Here's how the part is built. I have some questions about the finished solid (model axes, mm). A direction names the side the tool comes from. Coordinates: 2 decimals unless noted, no trailing zeros. Order: outer loops, then holes, each group sorted by start corner. A loop starts at its lowest first (then second) coordinate and runs counter-clockwise, first axis right, second up. Notation, with made-up numbers: (30, 12.5) - (70, 12.5) arc R21 ccw to (70, 24.5) - close; hole circle Ø11 at (-11, 34). An arc over 180 degrees is marked (long way). Answer as CSV lines item,"result". Start each with the question number.
Q1. Suppose I cut it at B-B (y = 9). Please give me the cut outline in (x, z).
Q2. Suppose I cut it at A-A (z = 29.5). Please give me the cut outline in (x, y).
Q3. Thinking about a two-plate mould opening in Z: for faces 3 (the face through (-12.545, -5, 19)), 4 (the face through (-13.559, 13.954, 35.976)), 5 (the face through (24.469, 13.954, 38.024)), 6 (the face through (5, -27, 3)), which applies, released by +Z, released by -Z, zero draft, split by the parting line, or undercut?
Q4. For pin 1 Ø1.2 at (y, z) = (-25.09, 37) entering from +X; pin 2 Ø2 at (x, y) = (5, -27) entering from +Z; pin 3 Ø11 at (x, y) = (14.5, -1) entering from +Z; pin 4 Ø4 at (x, z) = (0.5, 1) entering from +Y, each with a flat end and sliding along its axis, tell me the tip position at first contact or that it passes through.
Q5. Suppose I cut it at C-C (x = 19). Please give me the cut outline in (y, z).
Q6. For faces 1 (the face through (7, 16.909, -3)), 2 (the face through (5, -4, -2)), which set-ups out of +Z, -Z, +X, -X, +Y, -Y let a thin tool reach every point of the face, with its end or its side?
Q7. I need wall thicknesses on line 1 (Y direction, x = 24.6, z = 37); line 2 (X direction, y = 10, z = 22.5); line 3 (Z direction, x = 2.5, y = -15.5). Which ranges of each line are inside material? Lowest first, please.
from build123d import *

# Parameters (mm, degrees)
SKETCH_1_W           = 40
SKETCH_1_H           = 45
EXTRUDE_1_DEPTH      = 40
EXTRUDE_1_DEPTH_BACK = 5
SKETCH_2_W           = 36
SKETCH_2_H           = 37
CUT_EXTRUDE_1_DEPTH  = 50
SKETCH_3_R           = 1.025
CUT_EXTRUDE_2_DEPTH  = 2
SKETCH_4_R           = 1.025
CUT_EXTRUDE_3_DEPTH  = 2
SKETCH_5_W           = 36
SKETCH_5_H           = 5
CUT_EXTRUDE_4_DEPTH  = 43
FILLET_6_R           = 5
FILLET_7_R           = 5
FILLET_12_R          = 3
FILLET_13_R          = 3
FILLET_14_R          = 3
FILLET_15_R          = 3


with BuildPart() as part:
    # 草圖1 → 填料-伸長1 (new body, two sides)
    with BuildSketch(Plane.XY) as extrude_1_sk:
        with Locations((5.454545455, -5.590909091)):
            Rectangle(SKETCH_1_W, SKETCH_1_H)
    extrude(amount=EXTRUDE_1_DEPTH)
    extrude(extrude_1_sk.sketch, amount=-EXTRUDE_1_DEPTH_BACK)

    # 草圖2 → 除料-伸長1 (cut)
    with BuildSketch(Plane(origin=(0, 16.909090909, 0), x_dir=(1, 0, 0), z_dir=(0, 1, 0))):
        with Locations((5.454545455, -21.5)):
            Rectangle(SKETCH_2_W, SKETCH_2_H)
    extrude(amount=-CUT_EXTRUDE_1_DEPTH, mode=Mode.SUBTRACT)

    # 草圖3 → 除料-伸長2 (cut)
    with BuildSketch(Plane.ZY.offset(14.545454545)):
        with Locations((37, -25.090909091)):
            Circle(SKETCH_3_R)
        with Locations((37, 13.909090909)):
            Circle(SKETCH_3_R)
    extrude(amount=-CUT_EXTRUDE_2_DEPTH, mode=Mode.SUBTRACT)

    # 草圖4 → 除料-伸長3 (cut)
    with BuildSketch(Plane(origin=(25.454545455, 0, 0), x_dir=(0, 0, -1), z_dir=(1, 0, 0))):
        with Locations((-37, 13.909090909)):
            Circle(SKETCH_4_R)
        with Locations((-37, -25.090909091)):
            Circle(SKETCH_4_R)
    extrude(amount=-CUT_EXTRUDE_3_DEPTH, mode=Mode.SUBTRACT)

    # 草圖5 → 除料-伸長4 (cut)
    with BuildSketch(Plane(origin=(0, 16.909090909, 0), x_dir=(1, 0, 0), z_dir=(0, 1, 0))):
        with Locations((5.454545455, -0.5)):
            Rectangle(SKETCH_5_W, SKETCH_5_H)
    extrude(amount=-CUT_EXTRUDE_4_DEPTH, mode=Mode.SUBTRACT)

    # 圓角6
    fillet_6_edges = [part.edges().sort_by_distance(p)[0] for p in [
        (-14.545454545, -5.590909091, -5),
    ]]
    fillet(fillet_6_edges, radius=FILLET_6_R)

    # 圓角7
    fillet_7_edges = [part.edges().sort_by_distance(p)[0] for p in [
        (25.454545455, -5.590909091, -5),
    ]]
    fillet(fillet_7_edges, radius=FILLET_7_R)

    # 圓角12
    fillet_12_edges = [part.edges().sort_by_distance(p)[0] for p in [
        (-13.545454545, -28.090909091, 40),
    ]]
    fillet(fillet_12_edges, radius=FILLET_12_R)

    # 圓角13
    fillet_13_edges = [part.edges().sort_by_distance(p)[0] for p in [
        (24.454545455, -28.090909091, 40),
    ]]
    fillet(fillet_13_edges, radius=FILLET_13_R)

    # 圓角14
    fillet_14_edges = [part.edges().sort_by_distance(p)[0] for p in [
        (-13.545454545, 16.909090909, 40),
    ]]
    fillet(fillet_14_edges, radius=FILLET_14_R)

    # 圓角15
    fillet_15_edges = [part.edges().sort_by_distance(p)[0] for p in [
        (24.454545455, 16.909090909, 40),
    ]]
    fillet(fillet_15_edges, radius=FILLET_15_R)


solid = part.part
Here are the results:
1,outline,"(-14.55, 0) arc R5 ccw to (-9.55, -5) - (20.45, -5) arc R5 ccw to (25.45, 0) - (25.45, 40) - (23.45, 40) - (23.45, -2) - (-12.55, -2) - (-12.55, 40) - (-14.55, 40) - close"
2,outline,"(-14.55, -28.09) - (-12.55, -28.09) - (-12.55, 16.91) - (-14.55, 16.91) - close; (23.45, -28.09) - (25.45, -28.09) - (25.45, 16.91) - (23.45, 16.91) - close"
3,face 3,"zero draft"
3,face 4,"undercut"
3,face 5,"undercut"
3,face 6,"released by +Z"
4,pin 1,"passes through"
4,pin 2,"stops at z = 3"
4,pin 3,"stops at z = -2"
4,pin 4,"stops at y = -26.09"
5,outline,"(-28.09, -5) - (16.91, -5) - (16.91, -2) - (-26.09, -2) - (-26.09, 3) - (-28.09, 3) - close"
6,face 1,"+Z, -Z, +X, -X, +Y"
6,face 2,"+Z, +Y"
7,line 1,"y = -28.09 to -26.12, -24.07 to 12.88, 14.93 to 16.91"
7,line 2,"x = -14.55 to -12.55, 23.45 to 25.45"
7,line 3,"z = -5 to -2"
